Autodesk Inventor part; units mm, degrees
ref_plane "YZ Plane" through (0, 0, 0) normal (1, 0, 0) x (0, 1, 0)
ref_plane "XZ Plane" through (0, 0, 0) normal (0, 1, 0) x (-1, 0, 0)
ref_plane "XY Plane" through (0, 0, 0) normal (0, 0, 1) x (1, 0, 0)
ref_plane "Work Plane1" through (52.5141, 202.7033, 6.4479) normal (0, 0, -1) x (0, 1, 0)
sketch "Sketch1" plane through (52.5141, 202.7033, 6.4479) normal (0, 0, -1) x (0, 1, 0)
  circle A0 centre (-59.8114, -30.5) radius 2.95
  circle A1 centre (-38.8114, -18.3756) radius 2.95
  circle A2 centre (-38.8114, -42.6244) radius 2.95 construction
  circle A3 centre (-38.8114, -42.6244) radius 2.95
  line L0 (-38.8114, -42.6244) -> (-38.8114, -18.3756) construction
  line L1 (-38.8114, -18.3756) -> (-59.8114, -30.5) construction
  line L2 (-59.8114, -30.5) -> (-38.8114, -42.6244) construction
  line L3 (-63.9312, 9.5) -> (-63.9312, -70.5)
  line L4 (-63.9312, -70.5) -> (-33.9312, -70.5)
  line L5 (-33.9312, -70.5) -> (-33.9312, 9.5)
  line L6 (-33.9312, 9.5) -> (-63.9312, 9.5)
  line L7 (-63.9312, 9.5) -> (-33.9312, -70.5) construction
  line L8 (-63.9312, -70.5) -> (-33.9312, 9.5) construction
  point P0 (-202.7033, -52.5141)
  point P1 (-56.7146, -27.9576)
  point P2 (-59.6434, -27.5548)
  point P3 (-59.6434, -33.4452)
  dimension "d4" = 5.9
  dimension "d5" = 5.9
  dimension "d6" = 5.9
  dimension "d37" = 80
  dimension "d38" = 30
extrude "Extrusion1" add sketch "Sketch1" along normal blind 4
sketch "Sketch2" plane through (52.5141, 202.7033, 2.4479) normal (0, 0, -1) x (-1, 0, 0)
  circle A0 centre (42.6244, -38.8114) radius 2.95
  circle A1 centre (18.3756, -38.8114) radius 2.95
  circle A2 centre (30.5, -59.8114) radius 2.95
  line L0 (-9.5, -63.9312) -> (70.5, -63.9312)
  line L1 (70.5, -63.9312) -> (70.5, -33.9312)
  line L2 (70.5, -33.9312) -> (-9.5, -33.9312)
  line L3 (-9.5, -33.9312) -> (-9.5, -63.9312)
  point P0 (52.5141, -202.7033)
extrude "Extrusion2" add sketch "Sketch2" along normal blind 1.5 contours A0 | A1 | A2 | L3 L2 L1 L0
sketch "Skizze7" plane through (52.5141, 202.7033, 0.9479) normal (0, 0, -1) x (-1, 0, 0)
  line L0 (70.5, -63.9312) -> (70.5, -33.9312)
  line L1 (70.5, -33.9312) -> (-9.5, -33.9312)
  line L2 (-9.5, -33.9312) -> (-9.5, -63.9312)
  line L3 (-9.5, -63.9312) -> (70.5, -63.9312)
  line L4 (-8, -59.8091) -> (69, -59.8091)
  line L5 (69, -59.8091) -> (69, -33.8091)
  line L6 (69, -33.8091) -> (-8, -33.8091)
  line L7 (-8, -33.8091) -> (-8, -59.8091)
  line L8 (-8, -59.8091) -> (69, -33.8091) construction
  line L9 (69, -59.8091) -> (-8, -33.8091) construction
  line L10 (70.5, -33.9312) -> (-9.5, -33.9312)
  point P0 (52.5141, -202.7033)
  point P1 (30.5, -46.8091)
  point P2 (69, -33.9312)
  point P3 (-8, -33.9312)
  point P4 (69, -33.9312)
  dimension "d39" = 77
  dimension "d40" = 26
extrude "Extrusion7" add sketch "Skizze7" along normal blind 2 contours L3 L2 L1 L7 L4 L5 L0
ref_plane "Arbeitsebene2" through (22.0141, 138.7722, 6.4479) normal (-1, 0, 0) x (0, 0, 1)
properties part number "00_cellSTORM_v5_chiptray_slidesize"
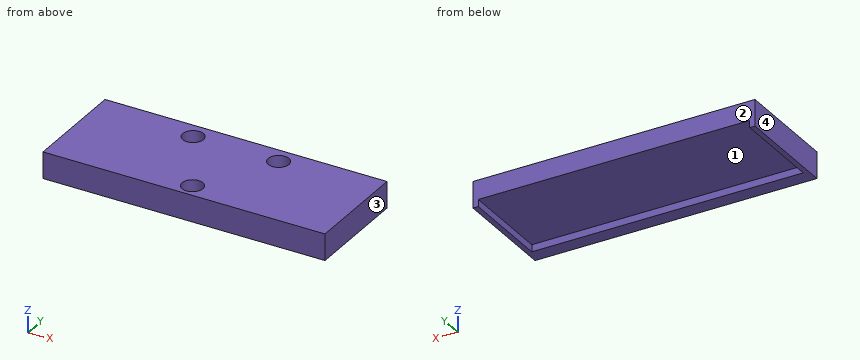
For this review, take the finished solid that the model builds, in its own axes (mm). Face numbers are marked on the shaded views. Give positions to 0.01 mm unless a question says otherwise; leave off trailing zeros. Order: outer loops, then holes, each group sorted by start corner. A loop starts at its lowest first (then second) coordinate and runs counter-clockwise, first axis right, second up. Notation, with made-up numbers: M 9.25,75.25 L 33.25,75.25 A17 ccw 33.25,104.25 Z; hole C 13,47.25 d9. An arc over 180 degrees is marked long. Answer in a Markdown table with one row per item. Add a question column.
(1) Consider section C-C on x = 40.5. State the section outline as (y, z) points.
(2) Mouldability with a two-part tool opening along X and no side actions: class the marked faces 1, 2, 3 and 4 as +X half, -X half, draft (parallel to the pull), parting line (faces both ways), or undercut.
(3) For pin 1 (5.5 mm diameter, centred on x = 9.89, y = 163.89, fed in from +Z); pin 2 (4 mm diameter, centred on x = 11.5, y = 161, fed in from -Z); pin 3 (1 mm diameter, centred on x = 22.5, z = 0, fed in from +Y), all flat-tipped, find the tip position at first contact; note any pin that passes through.
(4) Consider section B-B on z = 4.25. State the section outline as (x, y) points.
(5) Consider section D-D on y = 141.25. State the section outline as (x, z) points, and give its area (3 significant figures).
(6) Wall thickness on probe 1 along X at (y, z) = (152.75, 0.5); probe 2 along X at (y, z) = (161.5, 2.5); probe 3 along Z at (x, y) = (13.5, 159.25): over which ranges is each line inside the solid? List them lowest first. Write a range as [from, to].
(7) Consider section A-A on y = 157.25. State the section outline as (x, z) points, and give its area (3 significant figures).
Evaluation:
| question | item | result |
|---|---|---|
| 1 | outline | M 138.77,-1.05 L 142.89,-1.05 L 142.89,0.95 L 168.77,0.95 L 168.77,6.45 L 138.77,6.45 Z |
| 2 | face 1 | undercut |
| 2 | face 2 | draft |
| 2 | face 3 | +X half |
| 2 | face 4 | -X half |
| 3 | pin 1 | stops at z = 2.45 |
| 3 | pin 2 | stops at z = 0.95 |
| 3 | pin 3 | stops at y = 142.89 |
| 4 | outline | M -17.99,138.77 L 62.01,138.77 L 62.01,168.77 L -17.99,168.77 Z; hole C 9.89,163.89 d5.9; hole C 22.01,142.89 d5.9; hole C 34.14,163.89 d5.9 |
| 5 | outline | M -17.99,-1.05 L 62.01,-1.05 L 62.01,6.45 L 24.46,6.45 L 24.46,2.45 L 19.56,2.45 L 19.56,6.45 L -17.99,6.45 Z |
| 5 | area | 580 mm^2 |
| 6 | probe 1 | x = [-17.99, -16.49], [60.51, 62.01] |
| 6 | probe 2 | x = [-17.99, 8.16], [11.62, 32.41], [35.87, 62.01] |
| 6 | probe 3 | z = [0.95, 6.45] |
| 7 | outline | M -17.99,-1.05 L -16.49,-1.05 L -16.49,0.95 L 60.51,0.95 L 60.51,-1.05 L 62.01,-1.05 L 62.01,6.45 L -17.99,6.45 Z |
| 7 | area | 446 mm^2 |
